```python
from build123d import *

# Parameters (mm, degrees)
ESQUISSE1_W        = 366
ESQUISSE1_H        = 166
ESQUISSE1_R        = 2.2
ESQUISSE1_R_2      = 4.5
ESQUISSE1_R_3      = 6.5
BOSS_EXTRU_1_DEPTH = 3


with BuildPart() as part:
    # Esquisse1 → Boss.-Extru.1 (new body)
    with BuildSketch(Plane.XY):
        with Locations((183, 83)):
            Rectangle(ESQUISSE1_W, ESQUISSE1_H)
        with Locations((13, 153)):
            Circle(ESQUISSE1_R, mode=Mode.SUBTRACT)
        with Locations((13, 13)):
            Circle(ESQUISSE1_R, mode=Mode.SUBTRACT)
        with Locations((13, 83)):
            Circle(ESQUISSE1_R, mode=Mode.SUBTRACT)
        with Locations((173, 153)):
            Circle(ESQUISSE1_R, mode=Mode.SUBTRACT)
        with Locations((193, 83)):
            Circle(ESQUISSE1_R, mode=Mode.SUBTRACT)
        with Locations((173, 83)):
            Circle(ESQUISSE1_R, mode=Mode.SUBTRACT)
        with Locations((193, 153)):
            Circle(ESQUISSE1_R, mode=Mode.SUBTRACT)
        with Locations((353, 83)):
            Circle(ESQUISSE1_R, mode=Mode.SUBTRACT)
        with Locations((353, 13)):
            Circle(ESQUISSE1_R, mode=Mode.SUBTRACT)
        with Locations((353, 153)):
            Circle(ESQUISSE1_R, mode=Mode.SUBTRACT)
        with Locations((193, 13)):
            Circle(ESQUISSE1_R, mode=Mode.SUBTRACT)
        with Locations((173, 13)):
            Circle(ESQUISSE1_R, mode=Mode.SUBTRACT)
        with Locations((270.5, 83)):
            Circle(ESQUISSE1_R_2, mode=Mode.SUBTRACT)
        with Locations((95.5, 83)):
            Circle(ESQUISSE1_R_2, mode=Mode.SUBTRACT)
        with Locations((77.5, 101)):
            Circle(ESQUISSE1_R, mode=Mode.SUBTRACT)
        with Locations((113.5, 101)):
            Circle(ESQUISSE1_R, mode=Mode.SUBTRACT)
        with Locations((77.5, 65)):
            Circle(ESQUISSE1_R, mode=Mode.SUBTRACT)
        with Locations((113.5, 65)):
            Circle(ESQUISSE1_R, mode=Mode.SUBTRACT)
        with Locations((288.5, 65)):
            Circle(ESQUISSE1_R, mode=Mode.SUBTRACT)
        with Locations((252.5, 65)):
            Circle(ESQUISSE1_R, mode=Mode.SUBTRACT)
        with Locations((252.5, 101)):
            Circle(ESQUISSE1_R, mode=Mode.SUBTRACT)
        with Locations((288.5, 101)):
            Circle(ESQUISSE1_R, mode=Mode.SUBTRACT)
        with Locations((37, 49)):
            Circle(ESQUISSE1_R_3, mode=Mode.SUBTRACT)
        with Locations((61, 49)):
            Circle(ESQUISSE1_R_3, mode=Mode.SUBTRACT)
        with Locations((85, 49)):
            Circle(ESQUISSE1_R, mode=Mode.SUBTRACT)
        with Locations((13, 49)):
            Circle(ESQUISSE1_R, mode=Mode.SUBTRACT)
    extrude(amount=BOSS_EXTRU_1_DEPTH)


solid = part.part
```
Read the model definition and answer for the solid it produces. Units are mm, in the model's axes. Coordinates: 2 decimals unless noted, no trailing zeros. Loops run counter-clockwise (first coordinate to the right, second up) from the corner with the lowest first, then second, coordinate; pieces in that order, holes last.
(1) The mould has two halves that part along X. Classify faces 1 (the face through (274.792, 84.352, 1.479)), 2 (the face through (67, 46.5, 1.5)), 3 (the face through (180, 84, 3)): released by +X, released by -X, zero draft, split by the parting line, or undercut.
Solution:
face 1: undercut
face 2: undercut
face 3: zero draft
(2) Consider line 1 along Y through (x, z) = (353, 1.15); line 2 along Y through (x, z) = (13, 2.35); line 3 along X through (y, z) = (15, 1.7). Determine where each line is inside the solid, lowest interval first.
Solution:
line 1: y = 0 to 10.8, 15.2 to 80.8, 85.2 to 150.8, 155.2 to 166
line 2: y = 0 to 10.8, 15.2 to 46.8, 51.2 to 80.8, 85.2 to 150.8, 155.2 to 166
line 3: x = 0 to 12.08, 13.92 to 172.08, 173.92 to 192.08, 193.92 to 352.08, 353.92 to 366
(3) The part is cut by section A-A (x = 37). Determine the outline of the cut face in (y, z), and give its area (3 significant figures).
Solution:
outline: (0, 0) - (42.5, 0) - (42.5, 3) - (0, 3) - close; (55.5, 0) - (166, 0) - (166, 3) - (55.5, 3) - close
area: 459 mm2
(4) The part is cut by section B-B (x = 270.5). Determine the outline of the cut face in (y, z).
Solution:
outline: (0, 0) - (78.5, 0) - (78.5, 3) - (0, 3) - close; (87.5, 0) - (166, 0) - (166, 3) - (87.5, 3) - close
